```python
from build123d import *

# Parameters (mm, degrees)
F0_W     = 50.8
F0_H     = 101.6
F1_DEPTH = 152.4
F2_T     = -2.54
F3_W     = 51.070213
F3_H     = 101.830907
F4_DEPTH = 152.4


with BuildPart() as f1:
    # F0 (on Front) → F1 (new body)
    with BuildSketch(Plane.XZ):
        with Locations((-25.4, 5.327806)):
            Rectangle(F0_W, F0_H)
    extrude(amount=F1_DEPTH)

    # F2
    f2_openings = [f1.faces().sort_by_distance(p)[0] for p in [
        (-50.8, -76.2, 5.327806),
    ]]
    offset(amount=F2_T, openings=f2_openings)

    # F3 (on Front) → F4 (join)
    with BuildSketch(Plane.XZ):
        with Locations((25.535106, 4.952264)):
            Rectangle(F3_W, F3_H)
    extrude(amount=F4_DEPTH)


solid = f1.part
```
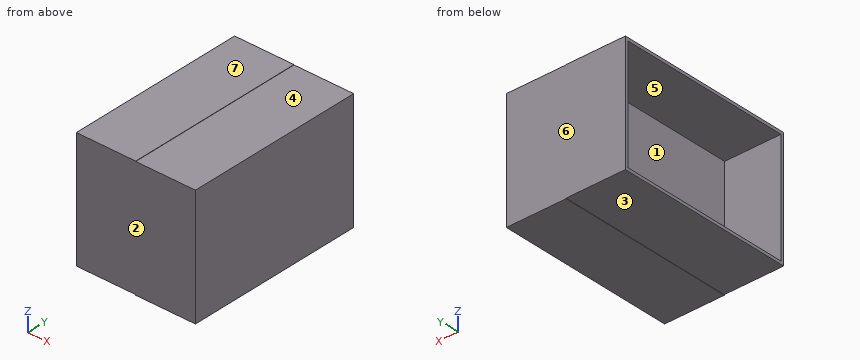
Read the model definition and answer for the solid it produces. Units are mm, in the model's axes. Face numbers are marked on the shaded views. A direction names the side the tool comes from. Give positions to 0.01 mm unless a question says otherwise; leave off trailing zeros. Order: outer loops, then holes, each group sorted by start corner. A loop starts at its lowest first (then second) coordinate and runs counter-clockwise, first axis right, second up.
(1) For a pull along Y with two mould halves and no side action, classify the marked faces 5, 6 and 7 as released by +Y, released by -Y, zero draft, split by the parting line, or undercut.
(2) Find section A-A (x = -41). Give the vertices of the cut face in (y, z), plus the area to 3 significant figures.
(3) Find section B-B (z = 25). Give the vertices of the cut face in (x, y), plus the area to 3 significant figures.
(4) Straight lines are drawn through the part: L1, parallel to Z at x = -43.5, y = -88.5; L2, parallel to Y at x = -14, z = 28; L3, parallel to X at y = -26.5, z = 22. For each, find the intervals that lie inside material, in ascending order.
(5) For the marked faces 1, 2, 3 and 4, determine the directions among +Z, -Z, +X, -X, +Y, -Y from which every point of the face is accessible in a straight line to the end or side of a thin tool.
(6) Find section C-C (y = -133). Give the vertices of the cut face in (x, z).
(7) Given pin 1 (5 mm diameter, centred on x = -38, z = 15.5, fed in from +Y); pin 2 (1.5 mm diameter, centred on y = -27.5, z = 26, fed in from -X); pin 3 (15 mm diameter, centred on x = -18.5, y = -94, fed in from -Z), each flat-ended and moving along its own axis, determine where each tip first touches the part or whether it passes through.
Result sheet:
1. face 5: undercut
1. face 6: released by +Y
1. face 7: zero draft
2. outline: (-152.4, -45.47) - (0, -45.47) - (0, 56.13) - (-152.4, 56.13) - close; hole (-149.86, -42.93) - (-2.54, -42.93) - (-2.54, 53.59) - (-149.86, 53.59) - close
2. area: 1,260 mm2
3. outline: (-50.8, -152.4) - (51.07, -152.4) - (51.07, 0) - (-50.8, 0) - (-50.8, -2.54) - (-2.54, -2.54) - (-2.54, -149.86) - (-50.8, -149.86) - close
3. area: 8,420 mm2
4. L1: z = -45.47 to -42.93, 53.59 to 56.13
4. L2: y = -152.4 to -149.86, -2.54 to 0
4. L3: x = -2.54 to 51.07
5. face 1: -X
5. face 2: +Z, -Z, +X, -X, -Y
5. face 3: -Z, -X, +Y, -Y
5. face 4: +Z, +X, +Y, -Y
6. outline: (-50.8, -45.47) - (0, -45.47) - (0, -45.96) - (51.07, -45.96) - (51.07, 55.87) - (0, 55.87) - (0, 56.13) - (-50.8, 56.13) - (-50.8, 53.59) - (-2.54, 53.59) - (-2.54, -42.93) - (-50.8, -42.93) - close
7. pin 1: stops at y = 0
7. pin 2: stops at x = -2.54
7. pin 3: stops at z = -45.47
